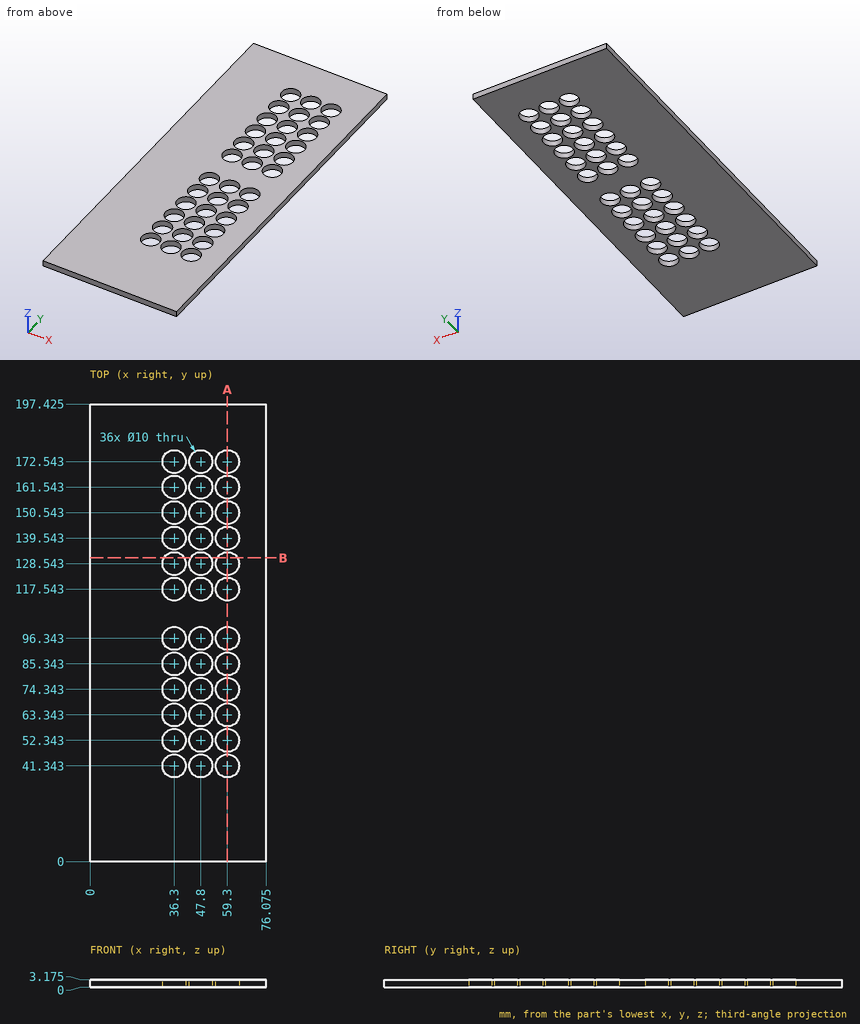
Job drawing, mm, ordinate dimensions from the low corner. One solid piece. Give positions to 0.01 mm unless a question says otherwise; leave off trailing zeros. Write each loop counter-clockwise with the first axis right and the second up, starting at its lowest first coordinate (ties: lowest second). Pieces come first, ordered by that corner, then holes. Notation, with made-up numbers: (84, 76.5) -> (88, 76.5) arc R26 cw to (88, 115.5) -> close; hole circle Ø11 at (-36.5, 57). An arc over 180 degrees is marked (long way). Return JSON: item names as keys, results as strings.
Item 1: Band-saw the part on A-A (x = 59.3). Give the number of separate pieces and of enclosed holes in the cut face, then the cut area to 3 significant figures.
Answer below:
{"separate pieces": "13", "enclosed holes": "0", "area": "246 mm2"}
Item 2: Drill centre lines: probe 1 along X at (y, z) = (38.5, 2) (1 decimal); probe 2 along X at (y, z) = (67, 0.3) (1 decimal). Where is each one in solid material? Low to high.
Answer below:
{"probe 1": "x = 0 to 32.2, 40.4 to 43.7, 51.9 to 55.2, 63.4 to 76.1", "probe 2": "x = 0 to 32.9, 39.7 to 44.4, 51.2 to 55.9, 62.7 to 76.1"}
Item 3: Drop a flat-ended pin along its axis: pin 1 (12 mm diameter, centred on x = 21, y = 78, fed in from -Z). Give the stop position or say it passes through.
Answer below:
{"pin 1": "stops at z = 0"}
Item 4: Band-saw the part on B-B (y = 131). List the corners of the cut face in (x, z) (1 decimal).
Answer below:
{"outline": "(0, 0) -> (31.9, 0) -> (31.9, 3.2) -> (0, 3.2) -> close; (40.7, 0) -> (43.4, 0) -> (43.4, 3.2) -> (40.7, 3.2) -> close; (52.2, 0) -> (54.9, 0) -> (54.9, 3.2) -> (52.2, 3.2) -> close; (63.7, 0) -> (76.1, 0) -> (76.1, 3.2) -> (63.7, 3.2) -> close"}
